Part model, mm, in its own coordinate system. Face numbers are marked on the shaded views. A direction names the side the tool comes from. Round coordinates to 2 decimals unless told otherwise and drop trailing zeros. Order: outer loops, then holes, each group sorted by start corner. A loop starts at its lowest first (then second) coordinate and runs counter-clockwise, first axis right, second up. Notation, with made-up numbers: M 75,-19.75 L 124,-19.75 A29 ccw 124,12.25 Z; hole C 72,41 d11. An arc over 180 degrees is marked long. Write each question's results on one line, items separated by ' | '. Start each with the question number.
1. Band-saw the part on A-A, the plane z = -44.1. List the corners of the cut face in (x, y).
2. Drop flat-ended pins along their axis: pin 1 Ø3 at (y, z) = (-8.75, -77) entering from -X; pin 2 Ø1.6 at (x, z) = (17, -20.5) entering from -Y; pin 3 Ø5 at (x, y) = (12.5, -1.5) entering from -Z; pin 4 Ø1 at (x, y) = (3.5, -8) entering from +Z. Give the stop position or say it passes through.
3. Band-saw the part on C-C, the plane x = -6. List the corners of the cut face in (y, z).
4. Band-saw the part on D-D, the plane z = -3.5. List the corners of the cut face in (x, y), then the cut area to 3 significant figures.
5. Which spindle directions (+Z, -Z, +X, -X, +Y, -Y) get a long thin tool onto all of the face, cutting with end or side? Do the marked faces 1 and 2. Say none if no direction does.
6. Probe L1, parallel to X at y = -0.5, z = -51.5; L2, parallel to Y at x = 17, z = -77; L3, parallel to Z at x = 16.85, y = -8.75. List the from-to ranges inside material, lowest first. Write a range as [from, to].
7. Band-saw the part on B-B, the plane z = -52.5. List the corners of the cut face in (x, y), then the cut area to 3 significant figures.
```python
from build123d import *

# Parameters (mm, degrees)
SKETCH1_R                = 0.95
BOSS_EXTRUDE1_DEPTH      = 18
FILLET1_R                = 2
CUT_EXTRUDE1_DEPTH       = 83.46596287
CUT_EXTRUDE1_DEPTH_BACK  = 83.46596287
SKETCH2_W                = 32
SKETCH2_H                = 82.41
BOSS_EXTRUDE2_DEPTH      = 18
BOSS_EXTRUDE2_DEPTH_BACK = 16
SKETCH3_R                = 3.75


with BuildPart() as part:
    # Sketch1 → Boss-Extrude1 (new, symmetric)
    with BuildSketch(Plane(origin=(0, 0, 0), x_dir=(0, 0, -1), z_dir=(1, 0, 0))):
        with BuildLine():
            Line((0, 3.13), (31.1, 3.13))
            Line((31.1, 3.13), (46.5, 1.782674582))
            Line((46.5, 1.782674582), (63, -0.639122384))
            Line((63, -0.639122384), (70.830854785, -5.891324783))
            ThreePointArc((70.830854785, -5.891324783), (73.097482442, -6.811154728), (75.542872081, -6.749855612))
            Line((75.542872081, -6.749855612), (76.479440337, -6.530221264))
            ThreePointArc((76.479440337, -6.530221264), (79.219778736, -8.229440337), (77.520559663, -10.969778736))
            Line((77.520559663, -10.969778736), (71.28999194, -13.416530703))
            ThreePointArc((71.28999194, -13.416530703), (68.724269269, -13.820147489), (66.228359009, -13.10162727))
            Line((66.228359009, -13.10162727), (61.611119998, -10.588406897))
            ThreePointArc((61.611119998, -10.588406897), (60.047418456, -10.001895705), (58.382627665, -9.86911952))
            Line((58.382627665, -9.86911952), (41.966210219, -10.855936181))
            Line((41.966210219, -10.855936181), (36.436012725, -11.188365046))
            ThreePointArc((36.436012725, -11.188365046), (35.406545304, -10.747772649), (35.143046066, -9.659428502))
            Line((35.143046066, -9.659428502), (35.942400407, -6.197044459))
            ThreePointArc((35.942400407, -6.197044459), (35.702698022, -5.137712345), (34.724437826, -4.665855641))
            Line((34.724437826, -4.665855641), (6.2959032, -4.665855641))
            Line((6.2959032, -4.665855641), (-0.7040968, -3.049778303))
            ThreePointArc((-0.7040968, -3.049778303), (-3.109879908, 0.354326059), (0, 3.13))
        make_face()
        Circle(SKETCH1_R, mode=Mode.SUBTRACT)
        with Locations((77, -8.75)):
            Circle(SKETCH1_R, mode=Mode.SUBTRACT)
        with Locations((44.1, -5.6)):
            Circle(SKETCH1_R, mode=Mode.SUBTRACT)
        with Locations((39.75, -8.75)):
            Circle(SKETCH1_R, mode=Mode.SUBTRACT)
    extrude(amount=BOSS_EXTRUDE1_DEPTH, both=True)

    # Fillet1
    # the kernel refuses this fillet: 2 mm, written as the material it takes off along each edge
    with BuildSketch(Plane(origin=(18.218304715, 3.13, -31.1), x_dir=(0, -0.08715574274766148, -0.9961946980917452), z_dir=(-1, 0, 0))) as fillet1_piece_1:
        with BuildLine():
            CenterArc((FILLET1_R * 0.0436609429085, FILLET1_R), FILLET1_R, 265, 5)
            Line((-FILLET1_R * 0.0434947998391, FILLET1_R * 0.00380530190825), (0, 0))
            Line((0, 0), (FILLET1_R * 0.0436609429085, 0))
        make_face()
    extrude(amount=36.436609429, mode=Mode.SUBTRACT)
    with BuildSketch(Plane(origin=(18.14621298, 1.782674582, -46.5), x_dir=(0, -0.14521967007723557, -0.9893994377513355), z_dir=(-1, 0, 0))) as fillet1_piece_2:
        with BuildLine():
            CenterArc((FILLET1_R * 0.0292425960983, FILLET1_R), FILLET1_R, 266.65, 3.35)
            Line((-FILLET1_R * 0.02919262642, FILLET1_R * 0.00170879761001), (0, 0))
            Line((0, 0), (FILLET1_R * 0.0292425960983, 0))
        make_face()
    extrude(amount=36.292425961, mode=Mode.SUBTRACT)
    with BuildSketch(Plane(origin=(19.131384491, -0.639122384, -63), x_dir=(0, -0.5570205743376995, -0.8304986934152874), z_dir=(-1, 0, 0))) as fillet1_piece_3:
        with BuildLine():
            CenterArc((FILLET1_R * 0.226276898255, FILLET1_R), FILLET1_R, 244.5, 25.5)
            Line((-FILLET1_R * 0.204234198553, FILLET1_R * 0.0974147156501), (0, 0))
            Line((0, 0), (FILLET1_R * 0.226276898255, 0))
        make_face()
    extrude(amount=38.262768983, mode=Mode.SUBTRACT)
    with BuildSketch(Plane(origin=(18.569678042, -4.665855641, -6.2959032), x_dir=(0, 0.22495105434386356, 0.9743700647852356), z_dir=(-1, 0, 0))) as fillet1_piece_4:
        with BuildLine():
            CenterArc((FILLET1_R * 0.113935608302, FILLET1_R), FILLET1_R, 257, 13)
            Line((-FILLET1_R * 0.111015446042, FILLET1_R * 0.0256299352148), (0, 0))
            Line((0, 0), (FILLET1_R * 0.113935608302, 0))
        make_face()
    extrude(amount=37.139356083, mode=Mode.SUBTRACT)

    # Sketch2 → Cut-Extrude1 (cut, two sides: drawn at the far end of the back side and taken through both)
    with BuildSketch(Plane(origin=(0, 0, 0), x_dir=(1, 0, 0), z_dir=(0, 1, 0)).offset(-CUT_EXTRUDE1_DEPTH_BACK)):
        with Locations((0, 38.075)):
            Rectangle(SKETCH2_W, SKETCH2_H)
    extrude(amount=CUT_EXTRUDE1_DEPTH + CUT_EXTRUDE1_DEPTH_BACK, mode=Mode.SUBTRACT)


with BuildPart() as cut_extrude1_piece_1:
    # of the separate pieces the step leaves, piece 1, a body of its own (cut_extrude1_pieces)
    add(part.part.solids().sort_by_distance((16, -13.416530703, -71.28999194))[0])



with BuildPart() as cut_extrude1_piece_2:
    # of the separate pieces the step leaves, piece 2, a body of its own (cut_extrude1_pieces)
    add(part.part.solids().sort_by_distance((-18, -13.416530703, -71.28999194))[0])


with BuildPart() as cut_extrude1_piece_1_1:
    add(cut_extrude1_piece_1.part)

    add(cut_extrude1_piece_2.part)  # Boss-Extrude2 merges Cut-Extrude1 piece 2
    # Sketch3 → Boss-Extrude2 (add, two sides: drawn at the far end of the back side and taken through both)
    with BuildSketch(Plane(origin=(0, 0, 0), x_dir=(0, 0, -1), z_dir=(1, 0, 0)).offset(-BOSS_EXTRUDE2_DEPTH_BACK)):
        with Locations((58.65, -5.75)):
            Circle(SKETCH3_R)
    extrude(amount=BOSS_EXTRUDE2_DEPTH + BOSS_EXTRUDE2_DEPTH_BACK)


solid = cut_extrude1_piece_1_1.part
```
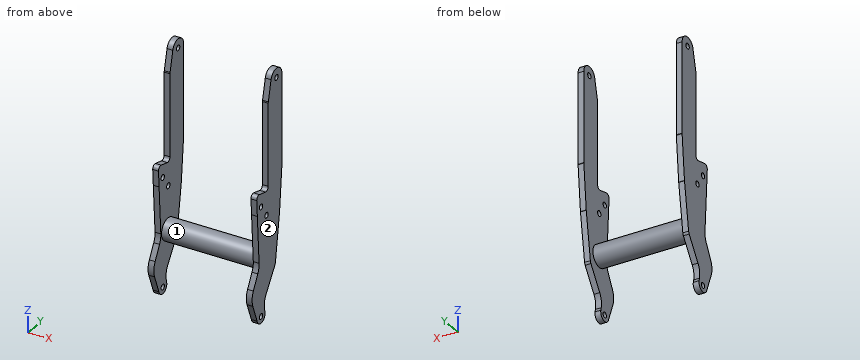
Solution:
1) outline: M -18,-10.73 L -16,-10.73 L -16,-6.55 L -18,-6.55 Z; M -18,-4.65 L -16,-4.65 L -16,1.99 L -18,1.99 Z; M 16,-10.73 L 18,-10.73 L 18,-6.55 L 16,-6.55 Z; M 16,-4.65 L 18,-4.65 L 18,1.99 L 16,1.99 Z
2) pin 1: x = -18 | pin 2: y = -4.67 | pin 3: z = -61.97 | pin 4: z = -55.33
3) outline: C -5.75,-58.65 d7.5
4) outline: M -18,-4.02 L -16,-4.02 L -16,3.13 L -18,3.13 Z; M 16,-4.02 L 18,-4.02 L 18,3.13 L 16,3.13 Z | area: 28.6 mm^2
5) face 1: none | face 2: +Z, -Z, +X, +Y, -Y
6) L1: [-18, -16], [16, 18] | L2: [-11.17, -9.7], [-7.8, -6.47] | L3: [-79.28, -77.95], [-76.05, -40.7], [-38.8, -35.35]
7) outline: M -18,-10.22 L -16,-10.22 L -16,0.9 L -18,0.9 Z; M 16,-10.22 L 18,-10.22 L 18,0.9 L 16,0.9 Z | area: 44.5 mm^2
